Design review of the part shown in the three views and the two pictorial views. Dimensions are in mm from the part's minimum x, y and z. A direction names the side the tool comes from. Round coordinates to 2 decimals unless told otherwise and drop trailing zeros. Order: outer loops, then holes, each group sorted by start corner. A loop starts at its lowest first (then second) coordinate and runs counter-clockwise, first axis right, second up.
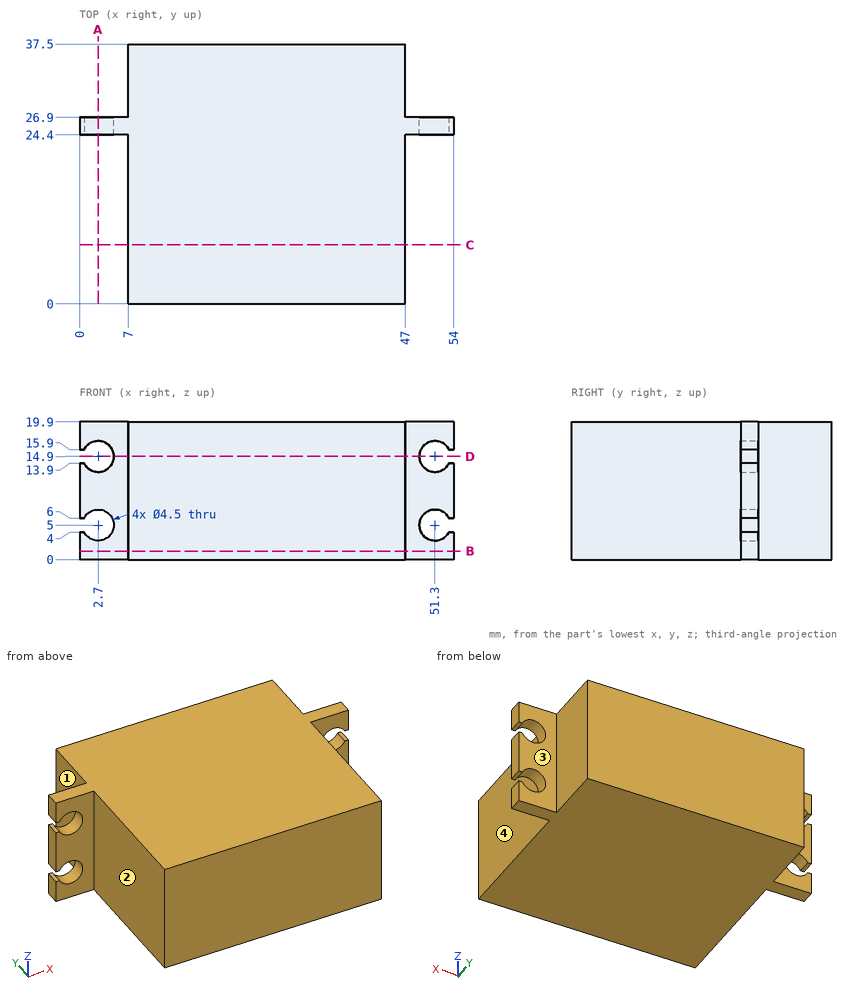
(1) Consider section D-D (z = 14.9). Write out the cut boundary in (x, y).
Data:
outline: (4.95, 24.4) - (7, 24.4) - (7, 0) - (47, 0) - (47, 24.4) - (49.05, 24.4) - (49.05, 26.9) - (47, 26.9) - (47, 37.5) - (7, 37.5) - (7, 26.9) - (4.95, 26.9) - close
(2) Consider section C-C (y = 8.5). Write out the cut boundary in (x, z).
Data:
outline: (7, 0) - (47, 0) - (47, 19.9) - (7, 19.9) - close
(3) To check wall thickness, follow probe 1 along Z at (x, y) = (2.7, 24.9); probe 2 along X at (y, z) = (25.95, 14.9); probe 3 along X at (y, z) = (32.5, 4.75). State the ranges of each line that lie inside material, in increasing order.
Data:
probe 1: z = 0 to 2.75, 7.25 to 12.65, 17.15 to 19.9
probe 2: x = 4.95 to 49.05
probe 3: x = 7 to 47
(4) Consider section B-B (z = 1.25). Write out the cut boundary in (x, y), and give its area (4 significant figures).
Data:
outline: (0, 24.4) - (7, 24.4) - (7, 0) - (47, 0) - (47, 24.4) - (54, 24.4) - (54, 26.9) - (47, 26.9) - (47, 37.5) - (7, 37.5) - (7, 26.9) - (0, 26.9) - close
area: 1,535 mm2
(5) Insertion check: pin 1 (2.5 mm diameter, centred on x = 51.3, z = 14.9, fed in from -Y); pin 2 (8.5 mm diameter, centred on y = 33, z = 10, fed in from -X); pin 3 (2 mm diameter, centred on y = 11.5, z = 3, fed in from +X); pin 4 (2 mm diameter, centred on x = 4, z = 12, fed in from +Y). Each pin has a flat end and moves straight along its axis. Give the tip position at first contact, or say it passes through.
Data:
pin 1: passes through
pin 2: stops at x = 7
pin 3: stops at x = 47
pin 4: stops at y = 26.9
(6) Consider section A-A (x = 2.7). Write out the cut boundary in (y, z).
Data:
outline: (24.4, 0) - (26.9, 0) - (26.9, 2.75) - (24.4, 2.75) - close; (24.4, 7.25) - (26.9, 7.25) - (26.9, 12.65) - (24.4, 12.65) - close; (24.4, 17.15) - (26.9, 17.15) - (26.9, 19.9) - (24.4, 19.9) - close
(7) For the marked faces 1, 2, 3 and 4, list the 3-axis set-ups (+Z, -Z, +X, -X, +Y, -Y) from which the entire face can be reached by the end or side of a thin tool; tool diameter is ignored.
Data:
face 1: +Z, -Z, -X, +Y
face 2: +Z, -Z, -X, -Y
face 3: +Z, -Z, +X, +Y
face 4: +Z, -Z, +X, -Y
